from build123d import *

# Parameters (mm, degrees)
PAD_DEPTH            = 12
SKETCH001_R          = 6
POCKET_DEPTH         = 12.001
PAD001_DEPTH         = 64
SKETCH003_W          = 40
SKETCH003_H          = 40
POCKET001_DEPTH      = 40.001
POCKET001_DEPTH_BACK = -40.001
POCKET002_DEPTH      = 64.001
SKETCH005_R          = 5
POCKET003_DEPTH      = 12.001


with BuildPart() as part:
    # Sketch → Pad (new body)
    with BuildSketch(Plane.XY):
        with BuildLine():
            Line((0, 40), (64, 40))
            Line((64, 40), (64, -40))
            Line((64, -40), (0, -40))
            ThreePointArc((0, -40), (-5.857864, -25.857864), (-20, -20))
            Line((-70, -20), (-20, -20))
            ThreePointArc((-70, 20), (-90, 0), (-70, -20))
            Line((-70, 20), (-19.999939, 20))
            ThreePointArc((-19.999939, 20), (-5.857843, 25.857886), (0, 40))
        make_face()
    extrude(amount=PAD_DEPTH)

    # Sketch001 (on DatumPlane) → Pocket (cut, through all)
    with BuildSketch(Plane.XY.offset(12)):
        with Locations((-70, 0)):
            Circle(SKETCH001_R)
    extrude(amount=-POCKET_DEPTH, mode=Mode.SUBTRACT)

    # Sketch002 → Pad001 (join)
    with BuildSketch(Plane.YZ):
        with BuildLine():
            Line((-40, 0), (40, 0))
            Line((40, 0), (40, 44.999965))
            ThreePointArc((40, 44.999965), (37.949747, 49.949747), (32.999965, 52))
            Line((32.999965, 52), (-33, 52))
            ThreePointArc((-33, 52), (-37.949747, 49.949748), (-40, 45))
            Line((-40, 45), (-40, 0))
        make_face()
    extrude(amount=PAD001_DEPTH)

    # Sketch003 → Pocket001 (cut, two sides)
    with BuildSketch(Plane.XZ) as pocket001_sk:
        with Locations((32, 32)):
            Rectangle(SKETCH003_W, SKETCH003_H)
    extrude(amount=-POCKET001_DEPTH, mode=Mode.SUBTRACT)
    extrude(pocket001_sk.sketch, amount=-POCKET001_DEPTH_BACK, mode=Mode.SUBTRACT)

    # Sketch004 → Pocket002 (cut, through all)
    with BuildSketch(Plane.YZ):
        with BuildLine():
            ThreePointArc((-25, 45), (-31, 39), (-25, 33))
            Line((-25, 33), (25, 33))
            ThreePointArc((25, 33), (31, 39), (25, 45))
            Line((-25, 45), (25, 45))
        make_face()
    extrude(amount=POCKET002_DEPTH, mode=Mode.SUBTRACT)

    # Sketch005 (on DatumPlane) → Pocket003 (cut, through all)
    with BuildSketch(Plane.XY.offset(12)):
        with Locations((32, 19.5)):
            Circle(SKETCH005_R)
        with Locations((32, -19.5)):
            Circle(SKETCH005_R)
    extrude(amount=-POCKET003_DEPTH, mode=Mode.SUBTRACT)


solid = part.part
Can you work these out from the model? Positions are in its coordinate system, mm. A direction names the side the tool comes from. Coordinates: 2 decimals unless noted, no trailing zeros. Loops run counter-clockwise (first coordinate to the right, second up) from the corner with the lowest first, then second, coordinate; pieces in that order, holes last. Notation, with made-up numbers: M 89,-5 L 125,-5 A23 cw 125,18 Z; hole C -2.5,63 d4. An arc over 180 degrees is marked long. Return JSON: item names as keys, results as strings. Group by question number.
Item 1: Imagine slicing it at C-C (x = 7.5). Please give me the cut outline in (y, z), and give its area (3 significant figures).
Item 2: If I drill on L1, parallel to Y at x = 32, z = 7; L2, parallel to X at y = 30, z = 49; L3, parallel to Z at x = -73, y = -17, over which ranges is the centre line in solid material (lowest first)? Write a range as from..to.
Item 3: Imagine slicing it at B-B (z = 9.5). Please give me the cut outline in (x, y), and give its area (3 significant figures).
Item 4: On a 3-axis mill with a long thin cutter (end or side, diameter ignored), from which of +Z, -Z, +X, -X, +Y, -Y can I reach the whole of each face in a straight line? I mean faces 5 (the flat face through (58, 0, 45)), 6 (the flat face through (-45, 20, 6)), 7 (the cylindrical face through (28, -22.5, 6.1)), 8 (the cylindrical face through (5.9, -37.9, 50)), 9 (the flat face through (-45, -20, 6)). Say none if no direction works.
Item 5: Imagine slicing it at A-A (y = 0). Please give me the cut outline in (x, z), and give its area (3 significant figures).
Item 6: Imagine slicing it at D-D (z = 43.5). Please give me the cut outline in (x, y), and give its area (3 significant figures).
Item 7: I'm going to push flat-ended pins straight in: pin 1 Ø8 at (x, y) = (41.5, -25) entering from +Z; pin 2 Ø10 at (x, z) = (-9, 13.5) entering from -Y; pin 3 Ø12 at (y, z) = (-12, 22) entering from -X. Where does each tip first touch, or does it pass through?
Item 8: Thinking about a two-plate mould opening in X: for faces 1 (the cylindrical face through (-5.703, -26.014, 5.916)), 2 (the flat face through (64, 1, 20)), 3 (the flat face through (32, 40, 7)), 4 (the flat face through (52, -1, 32)), which applies, released by +X, released by -X, zero draft, split by the parting line, or undercut?
Verdict:
{
 "1": {"outline": "M -40,0 L 40,0 L 40,45 A7 ccw 33,52 L -33,52 A7 ccw -40,45 Z; hole M -25,33 L 25,33 A6 ccw 25,45 L -25,45 A6 ccw Z", "area": "3,430 mm^2"},
 "2": {"L1": "y = -40..-24.5, -14.5..14.5, 24.5..40", "L2": "x = 0..12, 52..64", "L3": "z = 0..12"},
 "3": {"outline": "M -70,-20 L -20,-20 A20 cw 0,-40 L 64,-40 L 64,40 L 0,40 A20 cw -20,20 L -70,20 A20 ccw Z; hole C -70,0 d12; hole C 32,-19.5 d10; hole C 32,19.5 d10", "area": "8,450 mm^2"},
 "4": {"face 5": "+X, -X", "face 6": "+Z, -Z, -X, +Y", "face 7": "+Z, -Z", "face 8": "+Z, +X, -X, -Y", "face 9": "+Z, -Z, -X, -Y"},
 "5": {"outline": "M -90,0 L -76,0 L -76,12 L -90,12 Z; M -64,0 L 64,0 L 64,33 L 52,33 L 52,12 L 12,12 L 12,33 L 0,33 L 0,12 L -64,12 Z; M 0,45 L 12,45 L 12,52 L 0,52 Z; M 52,45 L 64,45 L 64,52 L 52,52 Z", "area": "2,380 mm^2"},
 "6": {"outline": "M 0,-40 L 12,-40 L 12,-28.97 L 0,-28.97 Z; M 0,28.97 L 12,28.97 L 12,40 L 0,40 Z; M 52,-40 L 64,-40 L 64,-28.97 L 52,-28.97 Z; M 52,28.97 L 64,28.97 L 64,40 L 52,40 Z", "area": "530 mm^2"},
 "7": {"pin 1": "stops at z = 12", "pin 2": "stops at y = -27.7", "pin 3": "stops at x = 0"},
 "8": {"face 1": "released by -X", "face 2": "released by +X", "face 3": "zero draft", "face 4": "undercut"}
}
